Part model, mm, in its own coordinate system. Face numbers are marked on the shaded views. A direction names the side the tool comes from. Round coordinates to 2 decimals unless told otherwise and drop trailing zeros. Order: outer loops, then holes, each group sorted by start corner. A loop starts at its lowest first (then second) coordinate and runs counter-clockwise, first axis right, second up. Notation, with made-up numbers: M 11.5,58.25 L 48.5,58.25 A14 cw 48.5,64.25 Z; hole C 46.5,66.5 d7. An arc over 180 degrees is marked long. Write each question's results on one line, items separated by ' | '. Start each with the question number.
1. Band-saw the part on A-A, the plane x = 27. List the corners of the cut face in (y, z).
2. Drop flat-ended pins along their axis: pin 1 Ø3 at (y, z) = (12.5, -17) entering from -X; pin 2 Ø8 at (y, z) = (75.5, 32.5) entering from -X; pin 3 Ø5 at (x, y) = (0, 25) entering from +Z; pin 4 Ø1.5 at (y, z) = (97.5, 11.5) entering from -X. Give the stop position or say it passes through.
3. Two-plate mould, pull along Z, no slides. Class the marked faces 3, 4 and 5: +Z half, -Z half, draft (parallel to the pull), parting line (faces both ways), or undercut.
4. Probe L1, parallel to Z at x = 0, y = -7; L2, parallel to Z at x = -11, y = 32; L3, parallel to Y at x = -45, z = -12.5. List the from-to ranges inside material, lowest first. Write a range as [from, to].
5. Band-saw the part on B-B, the plane y = 31. Give the number of separate pieces and of enclosed holes in the cut face, then the cut area to 3 significant figures.
6. Which spindle directions (+Z, -Z, +X, -X, +Y, -Y) get a long thin tool onto all of the face, cutting with end or side? Do the marked faces 1 and 2. Say none if no direction does.
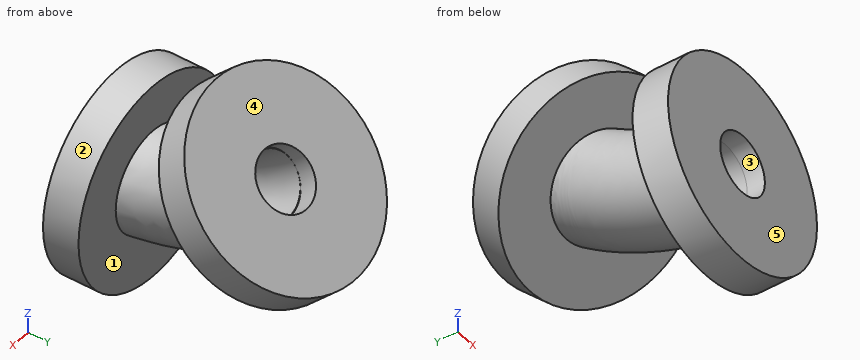
Solid Edge part; units mm, degrees
sketch "Sketch1" plane through (0, 0, 0) normal (1, 0, 0) x (0, 1, 0)
  arc A0 (0, 0) -> (69.7921, 28.3825) centre (-13.5476, 133.3134) ccw
sketch "Sketch2" plane through (0, 0, 0) normal (0, -1, 0) x (1, 0, 0)
  circle A0 centre (0, 0) radius 25
sweep "SweptProtrusion_2" add profiles "Sketch2" path "Sketch1"
sketch "Sketch3" plane through (0, 0, 0) normal (0, -1, 0) x (1, 0, 0)
  circle A0 centre (0, 0) radius 50
  circle A1 centre (0, 0) radius 15
extrude "ExtrudedProtrusion_6" add sketch "Sketch3" along normal blind 9
sketch "Sketch4" plane through (0, 0, 0) normal (0, -1, 0) x (1, 0, 0)
  circle A0 centre (0, 0) radius 50
  circle A1 centre (0, 0) radius 15
extrude "ExtrudedProtrusion_7" add sketch "Sketch4" against normal blind 9
mirror "Mirror1" about plane through (0, 36.9319, 9.1852) normal (0, 0.92633, 0.3767131) of "ExtrudedProtrusion_7"
mirror "Mirror2" about plane through (0, 36.9319, 9.1852) normal (0, 0.92633, 0.3767131) of "ExtrudedProtrusion_6"
sketch "Sketch5" plane through (0, 0, 0) normal (1, 0, 0) x (0, 1, 0)
  arc A0 (0, 0) -> (69.7921, 28.3825) centre (-13.5476, 133.3134) ccw
sketch "Sketch6" plane through (0, 0, 0) normal (0, -1, 0) x (1, 0, 0)
  circle A0 centre (0, 0) radius 15
sweep "SweptCutout_4" cut profiles "Sketch6" path "Sketch5"
Solution:
1) outline: M -9,-42.08 L 9,-42.08 L 9,42.08 L -9,42.08 Z; M 33.98,52.24 L 92.72,-8.04 L 105.61,4.52 L 46.87,64.8 Z
2) pin 1: x = -18.21 | pin 2: x = -50 | pin 3: z = 32.17 | pin 4: x = -39.48
3) face 3: undercut | face 4: +Z half | face 5: draft
4) L1: [-50, -15], [15, 50] | L2: [-16.26, -3.45], [18.13, 31.33], [54.27, 59.66] | L3: [-9, 9]
5) separate pieces: 2 | enclosed holes: 1 | area: 1,460 mm^2
6) face 1: none | face 2: -Y
